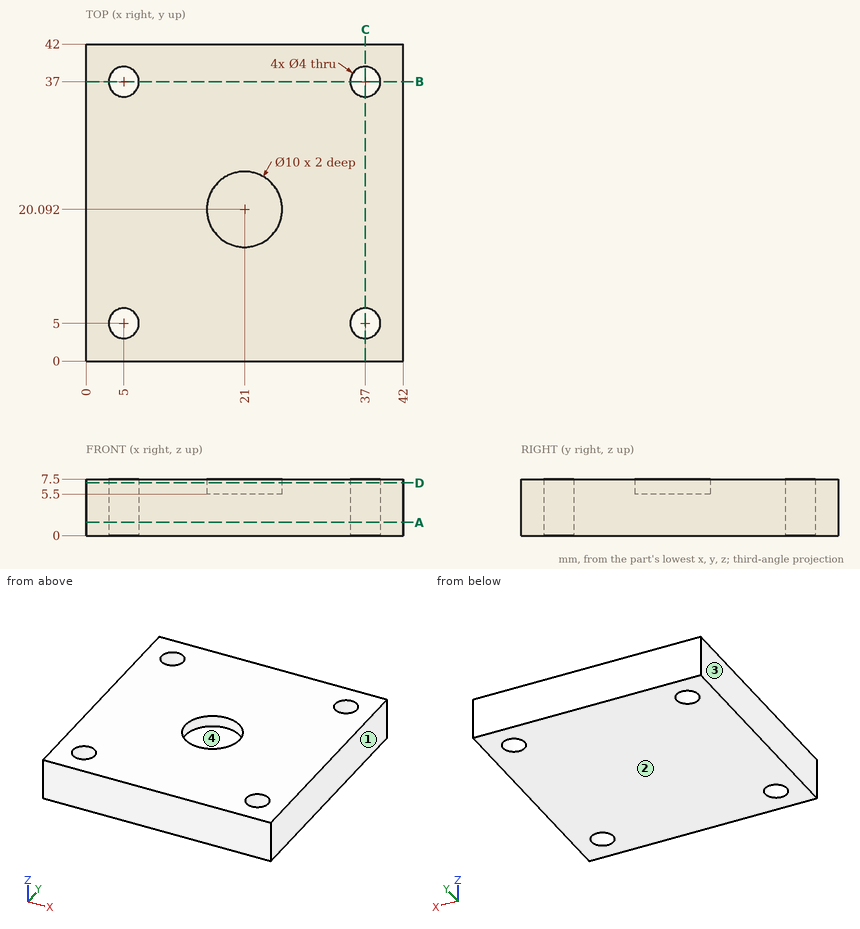
Print and shaded views of the part. All mm, measured from the part's lowest x, y and z. Coordinates: 2 decimals unless noted, no trailing zeros. Write each loop counter-clockwise with the first axis right and the second up, starting at its lowest first coordinate (ties: lowest second). Pieces come first, ordered by that corner, then holes. Notation, with made-up numbers: M 18.5,3.25 L 37.5,3.25 A29 cw 37.5,35.25 Z; hole C 62,40.25 d3. An arc over 180 degrees is marked long. Return JSON: item names as keys, results as strings.
1. Saw through at D-D, the plane z = 7. Write the cut outline in (x, y), then the cut area to 3 significant figures.
Determined:
{"outline": "M 0,0 L 42,0 L 42,42 L 0,42 Z; hole C 5,5 d4; hole C 5,37 d4; hole C 21,20.09 d10; hole C 37,5 d4; hole C 37,37 d4", "area": "1,640 mm²"}
2. Saw through at B-B, the plane y = 37. Write the cut outline in (x, z), then the cut area to 3 significant figures.
Determined:
{"outline": "M 0,0 L 3,0 L 3,7.5 L 0,7.5 Z; M 7,0 L 35,0 L 35,7.5 L 7,7.5 Z; M 39,0 L 42,0 L 42,7.5 L 39,7.5 Z", "area": "255 mm²"}
3. Saw through at A-A, the plane z = 1.75. Write the cut outline in (x, y).
Determined:
{"outline": "M 0,0 L 42,0 L 42,42 L 0,42 Z; hole C 5,5 d4; hole C 5,37 d4; hole C 37,5 d4; hole C 37,37 d4"}
4. Flat gauge pins, fed straight in: pin 1 Ø3.5 at (x, y) = (37, 37) entering from -Z; pin 2 Ø6.5 at (x, y) = (5, 5) entering from -Z; pin 3 Ø8 at (x, y) = (21, 20.09) entering from +Z. Where does each tip first touch, or does it go through?
Determined:
{"pin 1": "through", "pin 2": "z = 0", "pin 3": "z = 5.5"}
5. Pull direction X, two halves, no side cores. Call the marked faces 1, 2, 3 and 4: pulls with the +X half, pulls with the -X half, needs draft (parallel to the pull), parting line crosses it, or undercut.
Determined:
{"face 1": "pulls with the +X half", "face 2": "needs draft", "face 3": "pulls with the -X half", "face 4": "undercut"}
6. Probe L1, parallel to Y at x = 5, z = 4.5; L2, parallel to Y at x = 21, z = 6.6; L3, parallel to Y at x = 6.5, z = 2.5. List the from-to ranges inside material, lowest first.
Determined:
{"L1": "0 to 3, 7 to 35, 39 to 42", "L2": "0 to 15.09, 25.09 to 42", "L3": "0 to 3.68, 6.32 to 35.68, 38.32 to 42"}
